For this review, take the finished solid that the model builds, in its own axes (mm). Round coordinates to 2 decimals unless told otherwise and drop trailing zeros. Order: outer loops, then holes, each group sorted by start corner. A loop starts at its lowest first (then second) coordinate and runs counter-clockwise, first axis right, second up. Notation, with made-up numbers: (-8.5, 24.5) -> (29.5, 24.5) arc R27 cw to (29.5, 48.5) -> close; hole circle Ø6 at (-40, 76). An arc over 180 degrees is marked (long way). Use a Markdown table: item, result. Add a question column.
1) Clearance check with a flat-ended pin moving along its axis: P1, Ø2, axis at x = -10.39, y = -6, coming from the -Z side. State where the tip first meets the part, or that it passes through.
2) Consider section A-A (z = 1.15). State the section outline as (x, y) points, plus the area to 3 significant figures.
3) Consider section B-B (y = -6). Give the number of separate pieces and of enclosed holes in the cut face, plus the area to 3 significant figures.
4) Wall thickness on line 1 along Y through (x, z) = (0, 2.35); line 2 along X through (y, z) = (-6, 0.95); line 3 along X through (y, z) = (-5.5, 2.4): over which ranges is each line inside the solid? List them lowest first. Write a range as [from, to].
5) Draft analysis for pull direction X (two halves, no side actions). For faces 1 (the face through (9.139, -14.334, 1.979)), 2 (the face through (11.14, -5.024, 1.824)), 3 (the face through (3, 0, 4)), state which applies: pulls with the +X half, pulls with the -X half, needs draft (parallel to the pull), parting line crosses it, or undercut.
Autodesk Inventor part; units mm, degrees
ref_plane "Work Plane1" through (0, 0, 4) normal (0, 0, 1) x (1, 0, 0)
ref_plane "YZ Plane" through (0, 0, 0) normal (1, 0, 0) x (0, 1, 0)
ref_plane "XZ Plane" through (0, 0, 0) normal (0, 1, 0) x (-1, 0, 0)
sketch "Sketch1" plane through (0, 0, 0) normal (0, 0, 1) x (1, 0, 0)
  circle A0 centre (0, 0) radius 17
  dimension "d0" = 34
extrude "Extrusion1" add sketch "Sketch1" along normal blind 4
sketch "Sketch2" plane through (0, 0, 0) normal (1, 0, 0) x (0, 1, 0)
  line L0 (17, 4) -> (-17, 4)
  line L1 (0, 4) -> (0.8, 4)
  line L2 (0, 4) -> (0, 3.5381)
  line L3 (0, 3.5381) -> (0.8, 4)
  line L4 (0, -0.8) -> (0, 4.8)
  point P0 (0, 0)
  dimension "d3" = 0.8
  dimension "d40" = 60
revolve "Revolution1" cut sketch "Sketch2" angle 360 about axis through (0, 0, -10) along (0, 0, 1)
ref_plane "Work Plane1" through (0, 0, 4) normal (0, 0, 1) x (1, 0, 0)
sketch "Sketch3" plane through (0, 0, 4) normal (0, 0, 1) x (1, 0, 0)
  circle A0 centre (0, 0) radius 12
  point P0 (0, 12)
  point P1 (-10.3923, -6)
  point P2 (10.3923, -6)
  dimension "d7" = 24
  dimension "d10" = 360
hole "Hole7" at (0, 12, 4) at (-10.3923, -6, 4) at (10.3923, -6, 4) direction (0, 0, -1) diameter 2.459 end through all
chamfer "Chamfer2" distance 0.3 angle 45 3 edges at (-10.3923, -4.7705, 4) (10.3923, -4.7705, 4) (0, 13.2295, 4)
chamfer "Chamfer3" distance 0.5 angle 45 2 edges at (-17, 0, 4) (-17, 0, 0)
sketch "Sketch4" plane through (0, 0, 4) normal (0, 0, 1) x (1, 0, 0)
  point P0 (-51.4403, -28.5545)
  point P1 (-61.8326, -46.5545)
  point P2 (-72.2249, -28.5545)
sketch "Sketch5" plane through (0, 0, 4) normal (0, 0, 1) x (1, 0, 0)
  point P0 (-51.4403, -28.5545)
  point P1 (-61.8326, -46.5545)
  point P2 (-72.2249, -28.5545)
sketch "Sketch6" plane through (0, 0, 4) normal (0, 0, 1) x (1, 0, 0)
  point P0 (-51.4403, -28.5545)
properties part number "podporka_pajaka" material "Aluminium 6061"
Results list:
| question | item | result |
|---|---|---|
| 1 | P1 | through |
| 2 | outline | circle Ø34 at (0, 0); hole circle Ø2.46 at (-10.39, -6); hole circle Ø2.46 at (0, 12); hole circle Ø2.46 at (10.39, -6) |
| 2 | area | 894 mm2 |
| 3 | separate pieces | 3 |
| 3 | enclosed holes | 0 |
| 3 | area | 107 mm2 |
| 4 | line 1 | [-17, 10.77], [13.23, 17] |
| 4 | line 2 | [-15.91, -11.62], [-9.16, 9.16], [11.62, 15.91] |
| 4 | line 3 | [-16.09, -11.52], [-9.27, 9.27], [11.52, 16.09] |
| 5 | face 1 | parting line crosses it |
| 5 | face 2 | undercut |
| 5 | face 3 | needs draft |
